Model file for the job. Use its own axes, mm. Face numbers are marked on the shaded views. A direction names the side the tool comes from. Coordinates: 2 decimals unless noted, no trailing zeros. Order: outer loops, then holes, each group sorted by start corner. A loop starts at its lowest first (then second) coordinate and runs counter-clockwise, first axis right, second up.
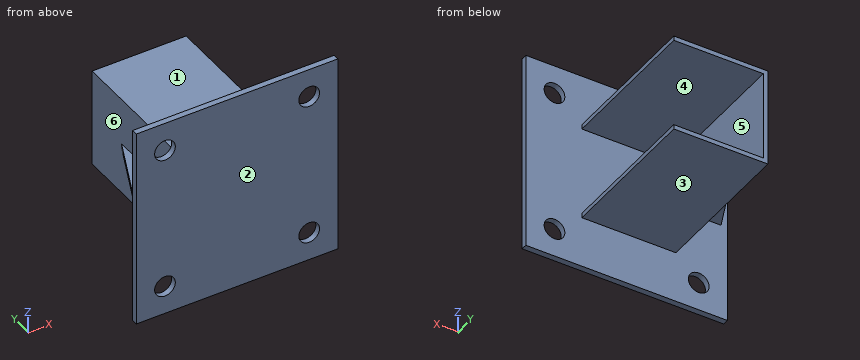
from build123d import *

# Parameters (mm, degrees)
SKETCH_1_W          = 136.3
SKETCH_1_H          = 136.3
EXTRUDE_1_DEPTH     = 4
EXTRUDE_2_DEPTH     = 100
CUT_EXTRUDE_1_DEPTH = 100
SKETCH_5_R          = 7
CUT_EXTRUDE_2_DEPTH = 100


with BuildPart() as part:
    # 草图1 → 凸台-拉伸1 (new body)
    with BuildSketch(Plane(origin=(0, 0, 0), x_dir=(1, 0, 0), z_dir=(0, 1, 0))):
        Rectangle(SKETCH_1_W, SKETCH_1_H)
    extrude(amount=EXTRUDE_1_DEPTH)

    # 草图2 → 凸台-拉伸2 (add)
    with BuildSketch(Plane(origin=(0, 4, 0), x_dir=(1, 0, 0), z_dir=(0, 1, 0))):
        Polygon((30.25, 30.25), (-30.25, 30.25), (-30.25, -30.25), (30.25, -30.25), (30.25, -33.35), (-33.35, -33.35), (-33.35, -1.55), (-63.85, -1.55), (-63.85, 1.55), (-33.35, 1.55), (-33.35, 33.35), (30.25, 33.35), align=None)
    extrude(amount=EXTRUDE_2_DEPTH)

    # 草图3 → 切除-拉伸1 (cut)
    with BuildSketch(Plane.XY.offset(1.55)):
        Polygon((-63.85, 4), (-33.35, 72), (-33.35, 104), (-63.85, 104), align=None)
    extrude(amount=-CUT_EXTRUDE_1_DEPTH, mode=Mode.SUBTRACT)

    # 草图5 → 切除-拉伸2 (cut)
    with BuildSketch(Plane(origin=(0, 4, 0), x_dir=(1, 0, 0), z_dir=(0, 1, 0))):
        with Locations(Location((48.75, 48.75, 0), (0, 0, 270))):
            Circle(SKETCH_5_R)
        with Locations(Location((48.75, -48.75, 0), (0, 0, 270))):
            Circle(SKETCH_5_R)
        with Locations(Location((-48.75, -48.75, 0), (0, 0, 270))):
            Circle(SKETCH_5_R)
        with Locations(Location((-48.75, 48.75, 0), (0, 0, 270))):
            Circle(SKETCH_5_R)
    extrude(amount=-CUT_EXTRUDE_2_DEPTH, mode=Mode.SUBTRACT)


solid = part.part
Q1. Cut at B-B, the plane z = -48.75. List the corners of the cut face in (x, y), plus the area to 3 significant figures.
Established:
outline: (-68.15, 0) - (-55.75, 0) - (-55.75, 4) - (-68.15, 4) - close; (-41.75, 0) - (41.75, 0) - (41.75, 4) - (-41.75, 4) - close; (55.75, 0) - (68.15, 0) - (68.15, 4) - (55.75, 4) - close
area: 433 mm2
Q2. Mould opens along Z. For the marked faces 1, 2, 3 and 4 say: pulls with the +Z half, pulls with the -Z half, needs draft (parallel to the pull), parting line crosses it, or undercut.
Established:
face 1: pulls with the +Z half
face 2: needs draft
face 3: pulls with the -Z half
face 4: undercut
Q3. Which spindle directions (+Z, -Z, +X, -X, +Y, -Y) get a long thin tool onto all of the face, cutting with end or side? Do the marked faces 5 and 6. Say none if no direction does.
Established:
face 5: +X, +Y
face 6: -X, +Y
Q4. Cut at D-D, the plane y = 95.5. List the corners of the cut face in (x, z).
Established:
outline: (-33.35, -33.35) - (30.25, -33.35) - (30.25, -30.25) - (-30.25, -30.25) - (-30.25, 30.25) - (30.25, 30.25) - (30.25, 33.35) - (-33.35, 33.35) - close
Q5. Cut at A-A, the plane x = 48.75. List the corners of the cut face in (y, z).
Established:
outline: (0, -68.15) - (4, -68.15) - (4, -55.75) - (0, -55.75) - close; (0, -41.75) - (4, -41.75) - (4, 41.75) - (0, 41.75) - close; (0, 55.75) - (4, 55.75) - (4, 68.15) - (0, 68.15) - close
Q6. Cut at C-C, the plane x = -17. List the corners of the cut face in (y, z).
Established:
outline: (0, -68.15) - (4, -68.15) - (4, -33.35) - (104, -33.35) - (104, -30.25) - (4, -30.25) - (4, 30.25) - (104, 30.25) - (104, 33.35) - (4, 33.35) - (4, 68.15) - (0, 68.15) - close
Q7. Probe line 1 (X direction, y = 1.1, z = -48.75); line 2 (Z direction, x = 48, y = 1); line 3 (Z direction, x = -26.5, y = 99). List the from-to ranges inside material, lowest first.
Established:
line 1: x = -68.15 to -55.75, -41.75 to 41.75, 55.75 to 68.15
line 2: z = -68.15 to -55.71, -41.79 to 41.79, 55.71 to 68.15
line 3: z = -33.35 to -30.25, 30.25 to 33.35
Q8. Drop flat-ended pins along their axis: P1, Ø4, axis at x = 9.5, z = -46.5, coming from the +Y side; P2, Ø1.6, axis at y = 54, z = 31.5, coming from the +X side; P3, Ø4, axis at y = 50, z = -15, coming from the -X side. Give the stop position or say it passes through.
Established:
P1: stops at y = 4
P2: stops at x = 30.25
P3: stops at x = -33.35
